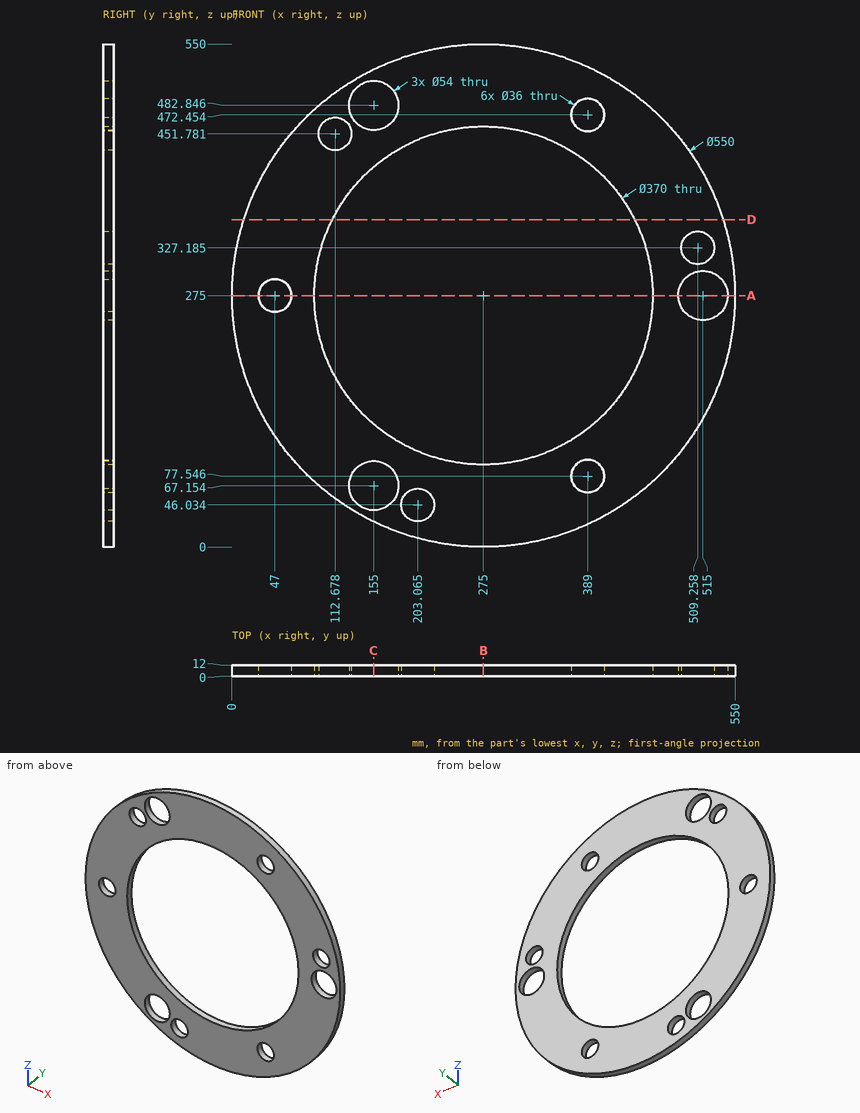
Can you work these out from the drawing? Everything is in mm from the part's minimum corner. Give positions to 0.01 mm unless a question says otherwise; leave off trailing zeros. Order: outer loops, then holes, each group sorted by start corner. A loop starts at its lowest first (then second) coordinate and runs counter-clockwise, first axis right, second up.
1. Suppose I cut it at D-D (z = 358). List the corners of the cut face in (x, y) for me (1 decimal).
2. I need wall thicknesses on L1, parallel to X at y = 4.5, z = 78.5 (1 decimal); L2, parallel to Z at x = 389, y = 3.5 (1 decimal); L3, parallel to X at y = 9.5, z = 73.5 (1 decimal). Which ranges of each line are inside material? Lowest first, please.
3. Suppose I cut it at A-A (z = 275). List the corners of the cut face in (x, y) for me.
4. Suppose I cut it at B-B (x = 275). List the corners of the cut face in (y, z) for me.
5. Suppose I cut it at C-C (x = 155). List the corners of the cut face in (y, z) for me.
6. Will these pins go through, and if not, where does the flat tip stop? P1, Ø4, axis at x = 437, y = 10, coming from the -Z side; P2, Ø6, axis at y = 10.5, z = 82.5, coming from the -X side (1 decimal); P3, Ø6, axis at x = 392, y = 1.5, coming from the -Z side.
Solved:
1. outline: (12.8, 0) - (109.7, 0) - (109.7, 12) - (12.8, 12) - close; (440.3, 0) - (537.2, 0) - (537.2, 12) - (440.3, 12) - close
2. L1: x = 82.6 to 130.5, 179.5 to 371, 407 to 467.4
2. L2: z = 24.7 to 59.5, 95.5 to 129.3, 420.7 to 454.5, 490.5 to 525.3
2. L3: x = 87.9 to 128.8, 181.2 to 371.5, 406.5 to 462.1
3. outline: (0, 0) - (29, 0) - (29, 12) - (0, 12) - close; (65, 0) - (90, 0) - (90, 12) - (65, 12) - close; (460, 0) - (488, 0) - (488, 12) - (460, 12) - close; (542, 0) - (550, 0) - (550, 12) - (542, 12) - close
4. outline: (0, 0) - (12, 0) - (12, 90) - (0, 90) - close; (0, 460) - (12, 460) - (12, 550) - (0, 550) - close
5. outline: (0, 27.56) - (12, 27.56) - (12, 40.15) - (0, 40.15) - close; (0, 94.15) - (12, 94.15) - (12, 134.2) - (0, 134.2) - close; (0, 415.8) - (12, 415.8) - (12, 455.85) - (0, 455.85) - close; (0, 509.85) - (12, 509.85) - (12, 522.44) - (0, 522.44) - close
6. P1: stops at z = 51.34
6. P2: stops at x = 75.7
6. P3: stops at z = 24.74
